Autodesk Inventor part; units mm, degrees
ref_plane "YZ Plane" through (0, 0, 0) normal (1, 0, 0) x (0, 1, 0)
ref_plane "XZ Plane" through (0, 0, 0) normal (0, 1, 0) x (-1, 0, 0)
ref_plane "XY Plane" through (0, 0, 0) normal (0, 0, 1) x (1, 0, 0)
sketch "Esboço1" plane through (0, 0, 0) normal (0, 0, 1) x (1, 0, 0)
  line L0 (101.6, -24.05) -> (-101.6, -24.05)
  line L1 (-101.6, -24.05) -> (-101.6, 24.05)
  line L2 (-101.6, 24.05) -> (101.6, 24.05)
  line L3 (101.6, 24.05) -> (101.6, -24.05)
  line L4 (101.6, -24.05) -> (-101.6, 24.05) construction
  line L5 (-101.6, -24.05) -> (101.6, 24.05) construction
  circle A0 centre (-88.9, 6.35) radius 2.5
  circle A1 centre (-88.9, -6.35) radius 2.5
  circle A2 centre (-88.9, 19.05) radius 2.5
  circle A3 centre (-88.9, -19.05) radius 2.5
  line L6 (0, 0) -> (0, 24.05)
  line L7 (-101.6, -24.05) -> (101.6, 24.05) construction
  line L8 (101.6, -24.05) -> (-101.6, 24.05) construction
  circle A4 centre (88.9, 6.35) radius 2.5
  circle A5 centre (88.9, -6.35) radius 2.5
  circle A6 centre (88.9, 19.05) radius 2.5
  circle A7 centre (88.9, -19.05) radius 2.5
  dimension "d0" = 203.2
  dimension "d1" = 5
  dimension "d2" = 12.7
  dimension "d3" = 12.7
  dimension "d4" = 12.7
  dimension "d5" = 12.7
  dimension "d6" = 5
  dimension "d7" = 5
extrude "Extrusão1" add sketch "Esboço1" along normal blind 5
sketch "Esboço2" plane through (0, 0, 0) normal (0, 0, -1) x (-1, 0, 0)
  line L0 (-101.6, 24.05) -> (101.6, 24.05)
  line L1 (12.7, -24.05) -> (-12.7, -24.05)
  line L2 (-12.7, -24.05) -> (-12.7, 24.05)
  line L3 (-12.7, 24.05) -> (12.7, 24.05)
  line L4 (12.7, 24.05) -> (12.7, -24.05)
  line L5 (12.7, -24.05) -> (-12.7, 24.05) construction
  line L6 (-12.7, -24.05) -> (12.7, 24.05) construction
  line L7 (17.7, -24.05) -> (-17.7, -24.05)
  line L8 (-17.7, -24.05) -> (-17.7, 24.05)
  line L9 (-17.7, 24.05) -> (17.7, 24.05)
  line L10 (17.7, 24.05) -> (17.7, -24.05)
  line L11 (17.7, -24.05) -> (-17.7, 24.05) construction
  line L12 (-17.7, -24.05) -> (17.7, 24.05) construction
  point P0 (0, 0)
  dimension "d10" = 25.4
  dimension "d11" = 5
extrude "Extrusão2" add sketch "Esboço2" along normal blind 25.4 contours L0 L2 L7 L8 | L0 L10 L7 L4
chamfer "Chanfro1" distance 25.4 angle 45 2 edges at (17.7, 0, 0) (-17.7, 0, 0)
equation "\"d3\" = d2"
equation "\"d4\" = d2"
equation "\"d7\" = d6"
properties part number "Chapa Guia - Elevador"
Design review of the part built by this model. Coordinates are the model's own, in mm. A direction names the side the tool comes from. Coordinates: 2 decimals unless noted, no trailing zeros. Order: outer loops, then holes, each group sorted by start corner. A loop starts at its lowest first (then second) coordinate and runs counter-clockwise, first axis right, second up. Notation, with made-up numbers: M 4.5,45 L 15.5,45 A21 cw 15.5,56 Z; hole C 69,26.5 d5. An arc over 180 degrees is marked long. Answer as a JSON object with one key per item and string values. Group by question number.
1) Wall thickness on L1, parallel to X at y = -6, z = 1; L2, parallel to Y at x = -88.9, z = 1.4; L3, parallel to Y at x = -88, z = 2.5: over which ranges is each line inside the solid? List them lowest first.
2) Add section A-A, the plane x = -88.9. Write out the cut boundary in (y, z).
3) Add section B-B, the plane y = -6.35. Count the separate pieces of the cut face and the enclosed holes in it, then the cut area to 3 significant figures.
4) Mouldability with a two-part tool opening along Y and no side actions: class faces 1 (the flat face through (0, 24.05, 3)), 2 (the cylindrical face through (86.916, 20.571, 2.465)), 3 (the flat face through (72, 0, 0)) as pulls with the +Y half, pulls with the -Y half, needs draft (parallel to the pull), parting line crosses it, or undercut.
5) Add section C-C, the plane z = -18.5. Write out the cut boundary in (x, y), then the cut area to 3 significant figures.
6) For pin 1 (5 mm diameter, centred on x = -49.5, y = 17, fed in from -Z); pin 2 (5 mm diameter, centred on y = -12, z = -5.5, fed in from -X); pin 3 (12.5 mm diameter, centred on y = 7, z = -16.5, fed in from -X), all flat-tipped, find the tip position at first contact; note any pin that passes through.
7) Tool access review of faces 4 (the cylindrical face through (-86.515, 5.599, 2.465)), 5 (the flat face through (12.7, 0, -13)), 6 (the flat face through (-73, 0, 0)): name each direction out of +Z, -Z, +X, -X, +Y, -Y from which nothing blocks a thin tool from reaching the whole face with its end or side.
Computed values:
{
 "1": {"L1": "x = -101.6 to -91.38, -86.42 to 86.42, 91.38 to 101.6", "L2": "y = -24.05 to -21.55, -16.55 to -8.85, -3.85 to 3.85, 8.85 to 16.55, 21.55 to 24.05", "L3": "y = -24.05 to -21.38, -16.72 to -8.68, -4.02 to 4.02, 8.68 to 16.72, 21.38 to 24.05"},
 "2": {"outline": "M -24.05,0 L -21.55,0 L -21.55,5 L -24.05,5 Z; M -16.55,0 L -8.85,0 L -8.85,5 L -16.55,5 Z; M -3.85,0 L 3.85,0 L 3.85,5 L -3.85,5 Z; M 8.85,0 L 16.55,0 L 16.55,5 L 8.85,5 Z; M 21.55,0 L 24.05,0 L 24.05,5 L 21.55,5 Z"},
 "3": {"separate pieces": "3", "enclosed holes": "0", "area": "1,870 mm^2"},
 "4": {"face 1": "pulls with the +Y half", "face 2": "undercut", "face 3": "needs draft"},
 "5": {"outline": "M -24.6,-24.05 L -12.7,-24.05 L -12.7,24.05 L -24.6,24.05 Z; M 12.7,-24.05 L 24.6,-24.05 L 24.6,24.05 L 12.7,24.05 Z", "area": "1,140 mm^2"},
 "6": {"pin 1": "stops at z = 0", "pin 2": "stops at x = -40.1", "pin 3": "stops at x = -32.85"},
 "7": {"face 4": "+Z, -Z", "face 5": "-Z, +Y, -Y", "face 6": "-Z, -X, +Y, -Y"}
}
